```python
from build123d import *

# Parameters (mm, degrees)
F0_R     = 25.6267942687
F0_R_2   = 20.2357295817
F3_DEPTH = 25.4
F5_R     = 19.18287463


with BuildPart() as f2:
    # F2: sweep along a path in F1
    with BuildLine(Plane.XY) as f2_path:
        ThreePointArc((-35.9766818583, -43.863195926), (-10.2970958453, -28.2399727094), (0, 0))
    # F0 (on Front) → F2 (sweep)
    with BuildSketch(Plane.XZ):
        Circle(F0_R)
        Circle(F0_R_2, mode=Mode.SUBTRACT)
    sweep(path=f2_path.line)

    # F3 (add): a face of the model
    f3_faces = [f2.faces().sort_by_distance(p)[0] for p in [
        (-41.4506358623, -19.570328804, 0),
    ]]
    extrude(f3_faces, amount=F3_DEPTH)

    # F4: F2 across plane


with BuildPart() as f2_1:
    add(f2.part)
    add(f2.part.mirror(Plane.XZ))

    # F7: sweep along a path in F6
    with BuildLine(Plane.XZ) as f7_path:
        ThreePointArc((65.4886364937, -18.9907755703), (34.213022198, -4.4306436508), (0, 0))
    # F5 (on Right) → F7 (sweep, cut)
    with BuildSketch(Plane.YZ):
        Circle(F5_R)
    sweep(path=f7_path.line, mode=Mode.SUBTRACT)


solid = f2_1.part
```
CAD build for the part. Positions are in the model's coordinates, mm. Round coordinates to 2 decimals unless told otherwise and drop trailing zeros. Write item = value, one per line. Start each with the question number.
Q1. Probe L1, parallel to Y at x = -39, z = -14.5; L2, parallel to Y at x = -22, z = 16; L3, parallel to Z at x = 8.5, y = -10. List the from-to ranges inside material, lowest first. Write a range as from..to.
Q2. Mould opens along X. For faces 1 (the cylindrical face through (-43.95, -65.445, -6.078)), 2 (the flat face through (-64.955, -30.811, -7.474)), 3 (the cylindrical face through (-49.41, 41.2, -25.02)) say: pulls with the +X half, pulls with the -X half, needs draft (parallel to the pull), parting line crosses it, or undercut.
Q3. Band-saw the part on A-A (z = -14). Count the separate pieces of the cut face and the enclosed holes in it, then the cut area to 3 significant figures.
Q4. Drop flat-ended pins along their axis: pin 1 (4 mm diameter, centred on x = -55, y = 47, fed in from -Z); pin 2 (2 mm diameter, centred on x = -44.5, z = -14, fed in from +Y); pin 3 (6 mm diameter, centred on x = -3.5, y = 16, fed in from +Z). Give the stop position or say it passes through.
Answers below:
q1.L1 = -66.2..-59.01, -30.08..-22.87, 22.87..30.08, 59.01..66.2
q1.L2 = -60.54..-52.29, -22.74..-9.29, 9.29..22.74, 52.29..60.54
q1.L3 = -23.79..-17.86, 17.86..23.79
q2.face_1 = undercut
q2.face_2 = pulls with the -X half
q2.face_3 = parting line crosses it
q3.separate_pieces = 3
q3.enclosed_holes = 0
q3.area = 2,180 mm2
q4.pin_1 = -25.63
q4.pin_2 = 68.46
q4.pin_3 = 25.63
